Autodesk Inventor part; units mm, degrees
ref_plane "YZ Plane" through (0, 0, 0) normal (1, 0, 0) x (0, 1, 0)
ref_plane "XZ Plane" through (0, 0, 0) normal (0, 1, 0) x (-1, 0, 0)
ref_plane "XY Plane" through (0, 0, 0) normal (0, 0, 1) x (1, 0, 0)
sketch "Sketch1" plane through (0, 0, 0) normal (0, 1, 0) x (-1, 0, 0)
  line L0 (22.5, 22.5) -> (-22.5, 22.5)
  line L1 (-22.5, 22.5) -> (-22.5, -22.5)
  line L2 (-22.5, -22.5) -> (22.5, -22.5)
  line L3 (22.5, -22.5) -> (22.5, 22.5)
  line L4 (22.5, 22.5) -> (-22.5, -22.5) construction
  line L5 (-22.5, 22.5) -> (22.5, -22.5) construction
  point P0 (0, 0)
  dimension "d0" = 45
  dimension "d1" = 45
extrude "Extrusion1" add sketch "Sketch1" along normal blind 27.5
sketch "Sketch2" plane through (0, 27.5, 0) normal (0, 1, 0) x (1, 0, 0)
  circle A0 centre (0, 0) radius 16
  dimension "d4" = 32
extrude "Extrusion2" add sketch "Sketch2" along normal blind 5
sketch "Sketch4" plane through (0, 0, 0) normal (0, -1, 0) x (1, 0, 0)
  point P0 (0, 0)
  point P1 (16.5, -16.5)
  point P2 (-16.5, -16.5)
  point P3 (-16.5, 16.5)
  point P4 (16.5, 16.5)
  dimension "d8" = 33
  dimension "d9" = 16.5
  dimension "d10" = 33
  dimension "d11" = 16.5
hole "Hole1" at (16.5, 0, -16.5) at (-16.5, 0, -16.5) at (-16.5, 0, 16.5) at (16.5, 0, 16.5) direction (0, 1, 0) diameter 4.917 depth 9.5 tip angle 118
sketch "Sketch3" plane through (0, 32.5, 0) normal (0, 1, 0) x (1, 0, 0)
  circle A0 centre (0, 0) radius 15
  dimension "d7" = 30
extrude "Extrusion3" cut sketch "Sketch3" against normal blind 28
sketch "Sketch5" plane through (0, 27.5, 0) normal (0, 1, 0) x (1, 0, 0)
  circle A0 centre (16.5, 16.5) radius 2.4585
  circle A1 centre (16.5, -16.5) radius 2.4585
  circle A2 centre (-16.5, -16.5) radius 2.4585
  circle A3 centre (-16.5, 16.5) radius 2.4585
  point P0 (0, 0)
hole "Hole2" at (16.5, 27.5, -16.5) at (16.5, 27.5, 16.5) at (-16.5, 27.5, 16.5) at (-16.5, 27.5, -16.5) direction (0, -1, 0) diameter 5 depth 10 tip angle 118
sketch "Sketch6" plane through (-22.5, 0, -22.5) normal (-1, 0, 0) x (0, 0, 1)
  line L0 (45, 0) -> (45, 27.5)
  line L1 (0, 27.5) -> (45, 27.5)
  point P0 (22.5, 0)
  point P1 (25, 12.5)
  dimension "d28" = 20
  dimension "d29" = 15
hole "Hole3" at (-22.5, 12.5, 2.5) direction (1, 0, 0) diameter 7.9175 depth 27.5375 tip angle 118
properties part number "2309HCMUTE-CDT23-NAP_DUOI"
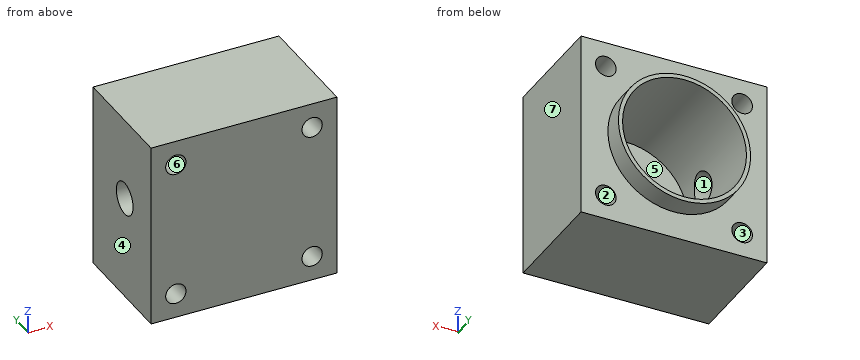
Model file for the job. Use its own axes, mm. Face numbers are marked on the shaded views. A direction names the side the tool comes from. Give positions to 0.01 mm unless a question says otherwise; leave off trailing zeros. Order: outer loops, then holes, each group sorted by start corner. A loop starts at its lowest first (then second) coordinate and runs counter-clockwise, first axis right, second up. Notation, with made-up numbers: (46, 28.25) - (99, 28.25) arc R27 ccw to (99, 44.25) - close; hole circle Ø10 at (-39, 10). An arc over 180 degrees is marked (long way). One line per item, written item: value.
Item 1: Slice it at B-B (z = 2.5). List the corners of the cut face in (x, y).
Response values:
outline: (-22.5, 0) - (22.5, 0) - (22.5, 27.5) - (15.8, 27.5) - (15.8, 32.5) - (14.79, 32.5) - (14.79, 4.5) - (-14.79, 4.5) - (-14.79, 8.54) - (-22.5, 8.54) - close; (-22.5, 16.46) - (-14.79, 16.46) - (-14.79, 32.5) - (-15.8, 32.5) - (-15.8, 27.5) - (-22.5, 27.5) - close
Item 2: Two-plate mould, pull along X, no slides. Class the marked faces 1, 2, 3 and 4: released by +X, released by -X, zero draft, split by the parting line, or undercut.
Response values:
face 1: zero draft
face 2: undercut
face 3: undercut
face 4: released by -X
Item 3: Slice it at D-D (x = 9). List the corners of the cut face in (y, z).
Response values:
outline: (0, -22.5) - (27.5, -22.5) - (27.5, -13.23) - (32.5, -13.23) - (32.5, -12) - (4.5, -12) - (4.5, 12) - (32.5, 12) - (32.5, 13.23) - (27.5, 13.23) - (27.5, 22.5) - (0, 22.5) - close
Item 4: Wall check: line 1 (Z direction, x = 16, y = 22); line 2 (X direction, y = 3.5, z = -16.5); line 3 (X direction, y = 3, z = -16). Give the ranges that are in metal, low to high.
Response values:
line 1: -22.5 to -18.95, -14.05 to 14.05, 18.95 to 22.5
line 2: -22.5 to -18.96, -14.04 to 14.04, 18.96 to 22.5
line 3: -22.5 to -18.91, -14.09 to 14.09, 18.91 to 22.5
Item 5: Slice it at A-A (y = 6.5). List the corners of the cut face in (x, z).
Response values:
outline: (-22.5, -22.5) - (22.5, -22.5) - (22.5, 22.5) - (-22.5, 22.5) - close; hole circle Ø4.92 at (-16.5, -16.5); hole circle Ø4.92 at (-16.5, 16.5); hole circle Ø30 at (0, 0); hole circle Ø4.92 at (16.5, -16.5); hole circle Ø4.92 at (16.5, 16.5)
Item 6: Tool access for the marked faces 5, 6 and 7: list every direction of +Z, -Z, +X, -X, +Y, -Y with a clear straight run to the whole face (end or side of a thin tool).
Response values:
face 5: +Y
face 6: -Y
face 7: +Z, -Z, +X, +Y, -Y
Item 7: Pin check, flat tips, straight feed: pin 1 Ø4 at (x, z) = (-5.5, 6) entering from +Y; pin 2 Ø4.5 at (x, z) = (-16.5, -16.5) entering from -Y; pin 3 Ø3 at (x, z) = (-16.5, 16.5) entering from -Y. Stop position of each tip, or through.
Response values:
pin 1: y = 4.5
pin 2: y = 9.63
pin 3: y = 10.08
Item 8: Slice it at C-C (y = 3). List the corners of the cut face in (x, z), then the cut area to 3 significant figures.
Response values:
outline: (-22.5, -22.5) - (22.5, -22.5) - (22.5, 22.5) - (-22.5, 22.5) - close; hole circle Ø4.92 at (-16.5, -16.5); hole circle Ø4.92 at (-16.5, 16.5); hole circle Ø4.92 at (16.5, -16.5); hole circle Ø4.92 at (16.5, 16.5)
area: 1,950 mm2
